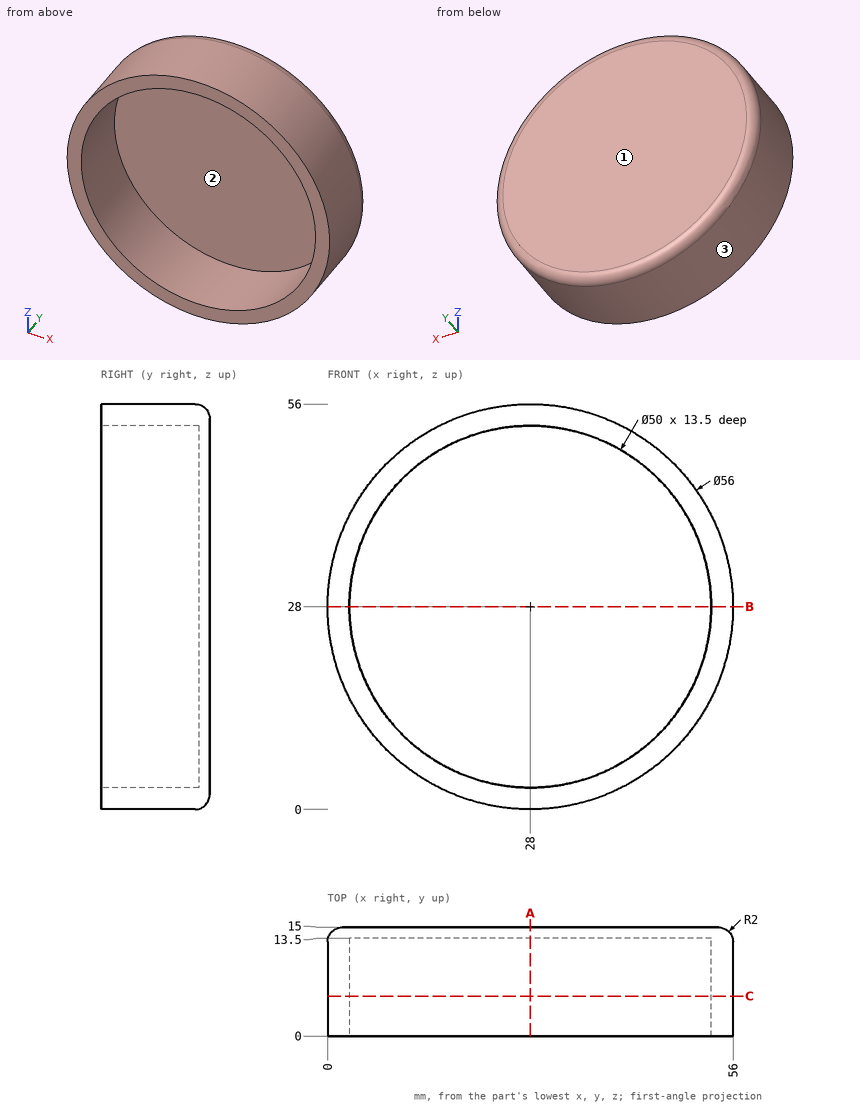
The drawing under review shows one solid part. Ordinate dimensions are in mm from its lowest x, y, z. Round coordinates to 2 decimals unless told otherwise and drop trailing zeros. Write each loop counter-clockwise with the first axis right and the second up, starting at its lowest first coordinate (ties: lowest second). Pieces come first, ordered by that corner, then holes. Notation, with made-up numbers: (52, 11.25) - (58, 11.25) arc R18 cw to (58, 40.25) - close; hole circle Ø9 at (-23.5, -21). An arc over 180 degrees is marked (long way). Use a Markdown table: item, result. Add a question column.
1. We need section A-A (x = 28). State the section outline as (y, z) points, then the cut area to 3 significant figures.
2. Wall thickness on probe 1 along Z at (x, y) = (28, 3.5); probe 2 along Y at (x, z) = (24.5, 7): over which ranges is each line inside the solid? List them lowest first.
3. Mouldability with a two-part tool opening along X and no side actions: class the marked faces 1, 2 and 3 as +X half, -X half, draft (parallel to the pull), parting line (faces both ways), or undercut.
4. We need section B-B (z = 28). State the section outline as (x, y) points.
5. We need section C-C (y = 5.5). State the section outline as (x, z) points, then the cut area to 3 significant figures.
6. Clearance check with flat-ended pins moving along their axes: pin 1 (6 mm diameter, centred on x = 35, y = 5.5, fed in from +Z); pin 2 (3 mm diameter, centred on x = 25.5, y = 8, fed in from -Z); pin 3 (1.5 mm diameter, centred on x = 40.5, y = 2, fed in from +Z). State where each tip first meets the part, or that it passes through.
Output:
| question | item | result |
|---|---|---|
| 1 | outline | (0, 0) - (13, 0) arc R2 ccw to (15, 2) - (15, 54) arc R2 ccw to (13, 56) - (0, 56) - (0, 53) - (13.5, 53) - (13.5, 3) - (0, 3) - close |
| 1 | area | 163 mm2 |
| 2 | probe 1 | z = 0 to 3, 53 to 56 |
| 2 | probe 2 | y = 13.5 to 15 |
| 3 | face 1 | draft |
| 3 | face 2 | undercut |
| 3 | face 3 | parting line |
| 4 | outline | (0, 0) - (3, 0) - (3, 13.5) - (53, 13.5) - (53, 0) - (56, 0) - (56, 13) arc R2 ccw to (54, 15) - (2, 15) arc R2 ccw to (0, 13) - close |
| 5 | outline | circle Ø56 at (28, 28); hole circle Ø50 at (28, 28) |
| 5 | area | 500 mm2 |
| 6 | pin 1 | stops at z = 55.71 |
| 6 | pin 2 | stops at z = 0.02 |
| 6 | pin 3 | stops at z = 53.42 |
